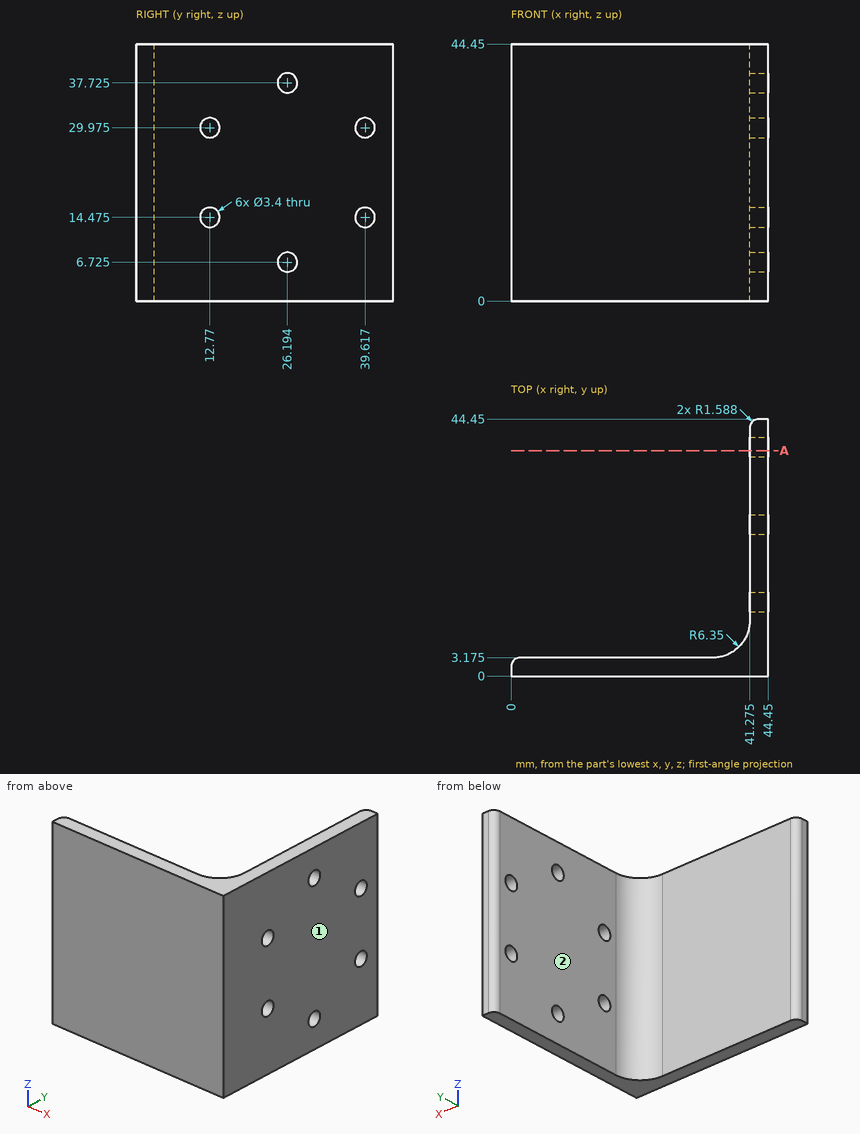
Design review of the part shown in the three views and the two pictorial views. Dimensions are in mm from the part's minimum x, y and z. A direction names the side the tool comes from. Coordinates: 2 decimals unless noted, no trailing zeros.
Item 1: For line 1 (Y direction, x = 10.5, z = 30.5) (1 decimal); line 2 (Y direction, x = 41.5, z = 18) (1 decimal); line 3 (X direction, y = 5, z = 36), list the stretches that pass through material, from the lowest coordinate up.
Item 2: For the marked faces 1 and 2, list the 3-axis set-ups (+Z, -Z, +X, -X, +Y, -Y) from which the entire face can be reached by the end or side of a thin tool; tool diameter is ignored.
Item 3: Take a section at A-A, the plane y = 39. Count the separate pieces of the cut face and the enclosed holes in it, then the cut area to 3 significant figures.
Item 4: For pin 1 Ø4 at (x, z) = (10.5, 8) entering from -Y; pin 2 Ø6 at (y, z) = (7.5, 9.5) entering from -X (1 decimal); pin 3 Ø2.5 at (y, z) = (26.19, 6.73) entering from -X; pin 4 Ø4 at (y, z) = (26.19, 37.72) entering from -X (1 decimal), all flat-tipped, find the tip position at first contact; note any pin that passes through.
The answers:
1. line 1: y = 0 to 3.2
1. line 2: y = 0 to 43.7
1. line 3: x = 39.38 to 44.45
2. face 1: +Z, -Z, +X, +Y, -Y
2. face 2: +Z, -Z, -X, +Y
3. separate pieces: 3
3. enclosed holes: 0
3. area: 121 mm2
4. pin 1: stops at y = 0
4. pin 2: stops at x = 38.8
4. pin 3: passes through
4. pin 4: stops at x = 41.3
